from build123d import *

# Parameters (mm, degrees)
SKETCH1_R               = 0.5
BOSS_EXTRUDE1_DEPTH     = 1.4
SKETCH2_R               = 2.35
CUT_EXTRUDE1_DEPTH      = 1
SKETCH3_R               = 3.5
SKETCH3_R_2             = 2.45
BOSS_EXTRUDE2_DEPTH     = 2.5
SKETCH4_R               = 1.2
CUT_EXTRUDE2_DEPTH      = 20.282440198
SKETCH5_R               = 2.45
SKETCH5_R_2             = 1.2
BOSS_EXTRUDE3_DEPTH     = 0.1
SKETCH6_W               = 35.735260114
SKETCH6_H               = 17.672039004
CUT_EXTRUDE4_DEPTH      = 20.513392837
CUT_EXTRUDE5_DEPTH      = 18.980545042
CUT_EXTRUDE_START       = -1.4
CUT_EXTRUDE_1_OUTLINE_R = 0.5
CUT_EXTRUDE_1_DEPTH     = 1.4


# Read off the part's stored shape, not the designer's step: 切除-拉伸-薄壁1
with BuildPart() as part:
    # Sketch1 → Boss-Extrude1 (new body)
    with BuildSketch(Plane(origin=(0, 0, 0), x_dir=(1, 0, 0), z_dir=(0, 1, 0))):
        with BuildLine():
            Line((-15.2, 2), (-2, 2.95))
            Line((-2, 2.95), (-2, 6.35))
            ThreePointArc((-2, 6.35), (0, 8.35), (2, 6.35))
            Line((2, 6.35), (2, 3.5))
            Line((2, 3.5), (15.2, 2))
            ThreePointArc((15.2, 2), (17.2, 0), (15.2, -2))
            Line((15.2, -2), (2, -3.5))
            Line((2, -3.5), (2, -6.35))
            ThreePointArc((2, -6.35), (0, -8.35), (-2, -6.35))
            Line((-2, -6.35), (-2, -2.95))
            Line((-2, -2.95), (-15.2, -2))
            ThreePointArc((-15.2, -2), (-17.2, 0), (-15.2, 2))
        make_face()
        with Locations((0, 6.35)):
            Circle(SKETCH1_R, mode=Mode.SUBTRACT)
        with Locations((0, 4.55)):
            Circle(SKETCH1_R, mode=Mode.SUBTRACT)
        with Locations((0, -4.55)):
            Circle(SKETCH1_R, mode=Mode.SUBTRACT)
        with Locations((0, -6.35)):
            Circle(SKETCH1_R, mode=Mode.SUBTRACT)
        with Locations((-15.2, 0)):
            Circle(SKETCH1_R, mode=Mode.SUBTRACT)
        with Locations(Location((15.2, 0, 0), (0, 0, 270))):
            Circle(SKETCH1_R, mode=Mode.SUBTRACT)
        with Locations((-13.4, 0)):
            Circle(SKETCH1_R, mode=Mode.SUBTRACT)
        with Locations((-11.6, 0)):
            Circle(SKETCH1_R, mode=Mode.SUBTRACT)
        with Locations((-9.8, 0)):
            Circle(SKETCH1_R, mode=Mode.SUBTRACT)
        with Locations((-8, 0)):
            Circle(SKETCH1_R, mode=Mode.SUBTRACT)
        with Locations((-6.2, 0)):
            Circle(SKETCH1_R, mode=Mode.SUBTRACT)
        with Locations((-4.4, 0)):
            Circle(SKETCH1_R, mode=Mode.SUBTRACT)
        with Locations(Location((13.4, 0, 0), (0, 0, 270))):
            Circle(SKETCH1_R, mode=Mode.SUBTRACT)
        with Locations(Location((11.6, 0, 0), (0, 0, 270))):
            Circle(SKETCH1_R, mode=Mode.SUBTRACT)
        with Locations(Location((9.8, 0, 0), (0, 0, 270))):
            Circle(SKETCH1_R, mode=Mode.SUBTRACT)
        with Locations(Location((8, 0, 0), (0, 0, 270))):
            Circle(SKETCH1_R, mode=Mode.SUBTRACT)
        with Locations(Location((6.2, 0, 0), (0, 0, 270))):
            Circle(SKETCH1_R, mode=Mode.SUBTRACT)
        with Locations(Location((4.4, 0, 0), (0, 0, 270))):
            Circle(SKETCH1_R, mode=Mode.SUBTRACT)
    extrude(amount=BOSS_EXTRUDE1_DEPTH)

    # Sketch2 → Cut-Extrude1 (cut)
    with BuildSketch(Plane.XZ):
        with Locations(Location((0, 0, 0), (0, 0, 270))):
            Circle(SKETCH2_R)
    extrude(amount=-CUT_EXTRUDE1_DEPTH, mode=Mode.SUBTRACT)

    # Sketch3 → Boss-Extrude2 (add)
    with BuildSketch(Plane(origin=(0, 1.4, 0), x_dir=(1, 0, 0), z_dir=(0, 1, 0))):
        with Locations(Location((0, 0, 0), (0, 0, 57.731921145))):
            Circle(SKETCH3_R)
        with Locations(Location((0, 0, 0), (0, 0, 270))):
            Circle(SKETCH3_R_2, mode=Mode.SUBTRACT)
    extrude(amount=BOSS_EXTRUDE2_DEPTH)

    # Sketch4 → Cut-Extrude2 (cut, through all)
    with BuildSketch(Plane(origin=(0, 1.4, 0), x_dir=(1, 0, 0), z_dir=(0, 1, 0))):
        with Locations(Location((0, 0, 0), (0, 0, 270))):
            Circle(SKETCH4_R)
    extrude(amount=-CUT_EXTRUDE2_DEPTH, mode=Mode.SUBTRACT)

    # Sketch5 → Boss-Extrude3 (add)
    with BuildSketch(Plane(origin=(0, 1.4, 0), x_dir=(1, 0, 0), z_dir=(0, 1, 0))):
        with Locations(Location((0, 0, 0), (0, 0, 270))):
            Circle(SKETCH5_R)
        with Locations(Location((0, 0, 0), (0, 0, 270))):
            Circle(SKETCH5_R_2, mode=Mode.SUBTRACT)
    extrude(amount=BOSS_EXTRUDE3_DEPTH)

    # Sketch6 → Cut-Extrude4 (cut, through all)
    with BuildSketch(Plane.XZ):
        Rectangle(SKETCH6_W, SKETCH6_H)
        with BuildLine():
            Line((-1.868584713, -2.959457918), (-15.2, -2))
            ThreePointArc((-15.2, -2), (-17.2, 0), (-15.2, 2))
            Line((-15.2, 2), (-1.868584713, 2.959457918))
            ThreePointArc((-1.868584713, 2.959457918), (0, 3.5), (1.868584713, 2.959457918))
            Line((1.868584713, 2.959457918), (15.2, 2))
            ThreePointArc((15.2, 2), (17.2, 0), (15.2, -2))
            Line((15.2, -2), (1.868584713, -2.959457918))
            ThreePointArc((1.868584713, -2.959457918), (0, -3.5), (-1.868584713, -2.959457918))
        make_face(mode=Mode.SUBTRACT)
    extrude(amount=-CUT_EXTRUDE4_DEPTH, mode=Mode.SUBTRACT)

    # Sketch7 → Cut-Extrude5 (cut, through all)
    with BuildSketch(Plane.XZ):
        with BuildLine():
            Line((0, 3.5), (-17.731768104, 3.5))
            Line((-17.731768104, 3.5), (-17.731768104, -3.5))
            Line((-17.731768104, -3.5), (0, -3.5))
            ThreePointArc((0, -3.5), (-3.5, 0), (0, 3.5))
        make_face()
    extrude(amount=-CUT_EXTRUDE5_DEPTH, mode=Mode.SUBTRACT)

    # 切除-拉伸-薄壁1 outline → 切除-拉伸-薄壁1 (cut)
    with BuildSketch(Plane(origin=(0, 0, 0), x_dir=(-1, 0, 0), z_dir=(0, -1, 0)).offset(CUT_EXTRUDE_START)):
        with BuildLine():
            Line((-4.4, -2.777272727), (-4.4, -0.5))
            ThreePointArc((-4.4, -0.5), (-4.9, 0), (-4.4, 0.5))
            Line((-4.4, 0.5), (-4.4, 2.777272727))
            Line((-4.4, 2.777272727), (-15.2, 2))
            ThreePointArc((-15.2, 2), (-17.2, 0), (-15.2, -2))
            Line((-15.2, -2), (-4.4, -2.777272727))
        make_face()
        with Locations((-15.2, 0)):
            Circle(CUT_EXTRUDE_1_OUTLINE_R, mode=Mode.SUBTRACT)
        with Locations((-13.4, 0)):
            Circle(CUT_EXTRUDE_1_OUTLINE_R, mode=Mode.SUBTRACT)
        with Locations((-11.6, 0)):
            Circle(CUT_EXTRUDE_1_OUTLINE_R, mode=Mode.SUBTRACT)
        with Locations((-9.8, 0)):
            Circle(CUT_EXTRUDE_1_OUTLINE_R, mode=Mode.SUBTRACT)
        with Locations((-8, 0)):
            Circle(CUT_EXTRUDE_1_OUTLINE_R, mode=Mode.SUBTRACT)
        with Locations((-6.2, 0)):
            Circle(CUT_EXTRUDE_1_OUTLINE_R, mode=Mode.SUBTRACT)
    extrude(amount=CUT_EXTRUDE_1_DEPTH, mode=Mode.SUBTRACT)


solid = part.part
Check sheet for the modelled part. Datum: model origin and axes. Units: mm. A direction names the side the tool comes from. Round coordinates to 2 decimals unless told otherwise and drop trailing zeros. Loops run counter-clockwise (first coordinate to the right, second up) from the corner with the lowest first, then second, coordinate; pieces in that order, holes last.
1. Sectioned sample at B-B on y = 1.1. Record the boundary of the cut face in (x, z).
2. Set-up check for faces 1 (the flat face through (1, 1, 1)), 2 (the flat face through (4.4, 1, 2)), 3 (the flat face through (3.7, 1.4, 0)), 4 (the cylindrical face through (0.736, 2.683, 2.337)): record each of +Z, -Z, +X, -X, +Y, -Y from which the full face is reachable in a straight line by a thin tool's end or side.
3. Mould release check, pull along Z, two halves, no side actions. Record for faces 5 (the flat face through (4.4, 1, -2)), 6 (the flat face through (3.12, 0.69, 2.87)), 7 (the flat face through (3.152, 0.69, -2.867)), 8 (the cylindrical face through (0.71, 0.49, -2.24)): released by +Z, released by -Z, zero draft, split by the parting line, or undercut.
4. Sectioned sample at A-A on z = 0. Record the boundary of the cut face in (x, y).
5. Sectioned sample at C-C on x = 4.25. Record the boundary of the cut face in (y, z), and give its area (3 significant figures).
6. Sectioned sample at D-D on x = 3.25. Record the boundary of the cut face in (y, z), and give its area (3 significant figures).
7. Scan lines: probe 1 along X at (y, z) = (3.05, 0); probe 2 along X at (y, z) = (0.3, 0); probe 3 along Z at (x, y) = (-0.25, 1.9). Record each from-to range of solid material in increasing order.
8. Gauge pin test, flat ends, axial feed: pin 1 Ø1.4 at (x, z) = (0, 0) entering from -Y; pin 2 Ø3 at (x, z) = (0, 0) entering from -Y; pin 3 Ø1 at (x, y) = (1.5, 1.5) entering from -Z; pin 4 Ø3 at (x, z) = (0, 0) entering from +Y. Record the tip position at first contact, or that the pin passes through.
Recorded:
1. outline: (1.87, -2.96) - (4.4, -2.78) - (4.4, -0.5) arc R0.5 cw to (4.4, 0.5) - (4.4, 2.78) - (1.87, 2.96) arc R3.5 ccw (long way) to start; hole circle Ø2.4 at (0, 0)
2. face 1: -Y
2. face 2: +Z, -Z, +X, +Y, -Y
2. face 3: +X, +Y
2. face 4: +Y
3. face 5: zero draft
3. face 6: released by +Z
3. face 7: released by -Z
3. face 8: undercut
4. outline: (-3.5, 0) - (-2.35, 0) - (-2.35, 1) - (-1.2, 1) - (-1.2, 1.5) - (-2.45, 1.5) - (-2.45, 3.9) - (-3.5, 3.9) - close; (1.2, 1) - (2.35, 1) - (2.35, 0) - (3.9, 0) - (3.9, 1.4) - (3.5, 1.4) - (3.5, 3.9) - (2.45, 3.9) - (2.45, 1.5) - (1.2, 1.5) - close
5. outline: (0, -2.79) - (1.4, -2.79) - (1.4, -0.48) - (0, -0.48) - close; (0, 0.48) - (1.4, 0.48) - (1.4, 2.79) - (0, 2.79) - close
5. area: 6.47 mm2
6. outline: (0, -2.86) - (1.4, -2.86) - (1.4, -1.3) - (3.9, -1.3) - (3.9, 1.3) - (1.4, 1.3) - (1.4, 2.86) - (0, 2.86) - close
6. area: 14.5 mm2
7. probe 1: x = -3.5 to -2.45, 2.45 to 3.5
7. probe 2: x = -3.5 to -2.35, 2.35 to 3.9
7. probe 3: z = -3.49 to -2.44, 2.44 to 3.49
8. pin 1: passes through
8. pin 2: stops at y = 1
8. pin 3: stops at z = -3.35
8. pin 4: stops at y = 1.5
